from build123d import *

# Parameters (mm, degrees)
PLATE_DEPTH             = 5.08
BOLTHOLES_REACH         = 38.278
SKETCH15_R              = 2.413
UPRIGHT_START           = 67.31
UPRIGHT_DEPTH           = 67.31
UPRIGHT_BOLTHOLES_REACH = 80.133
SKETCH17_R              = 2.54
SKETCH17_R_2            = 2.667
NUT_HOLE_START          = -2.54
NUT_HOLE_DEPTH          = 5.715


with BuildPart() as part:
    # Sketch2 → plate (new body)
    with BuildSketch(Plane(origin=(0, 0, 0), x_dir=(1, 0, 0), z_dir=(0, 1, 0))):
        with BuildLine():
            Line((-15.24, -20.32), (-15.24, -9.8425))
            Line((-15.24, -9.8425), (-3.81, -9.8425))
            Line((-3.81, -9.8425), (-3.81, 9.8425))
            Line((-3.81, 9.8425), (-15.24, 9.8425))
            Line((-15.24, 9.8425), (-15.24, 20.32))
            ThreePointArc((-15.24, 20.32), (25.4, 0), (-15.24, -20.32))
        make_face()
    extrude(amount=PLATE_DEPTH)

    # Sketch15 → boltholes (cut, up to next)
    with BuildSketch(Plane.XZ, mode=Mode.PRIVATE) as boltholes_sk1:
        with Locations(Location((8.89, 13.97, 0), (0, 0, 270))):
            Circle(SKETCH15_R)
    boltholes_tool1 = extrude(boltholes_sk1.sketch, amount=-BOLTHOLES_REACH, mode=Mode.PRIVATE) & part.part
    # Sketch15 → boltholes (cut, up to next)
    with BuildSketch(Plane.XZ, mode=Mode.PRIVATE) as boltholes_sk2:
        with Locations(Location((8.89, -13.97, 0), (0, 0, 270))):
            Circle(SKETCH15_R)
    boltholes_tool2 = extrude(boltholes_sk2.sketch, amount=-BOLTHOLES_REACH, mode=Mode.PRIVATE) & part.part
    add(boltholes_tool1.solids().sort_by_distance((8.89, 0, 13.97))[0], mode=Mode.SUBTRACT)
    add(boltholes_tool2.solids().sort_by_distance((8.89, 0, -13.97))[0], mode=Mode.SUBTRACT)

    # Sketch16 → upright (add)
    with BuildSketch(Plane.XZ.offset(UPRIGHT_START)):
        with BuildLine():
            Line((15.24, 20.32), (15.24, -20.32))
            ThreePointArc((15.24, -20.32), (21.962512448, -12.759625659), (25.200781238, -3.175))
            Line((25.200781238, -3.175), (22.025781238, -3.175))
            Line((22.025781238, -3.175), (22.025781238, 3.175))
            Line((22.025781238, 3.175), (25.200781238, 3.175))
            ThreePointArc((25.200781238, 3.175), (21.962512448, 12.759625659), (15.24, 20.32))
        make_face()
    extrude(amount=-UPRIGHT_DEPTH)

    # Sketch17 → upright_boltholes (cut, up to next)
    with BuildSketch(Plane.ZY.offset(-15.24), mode=Mode.PRIVATE) as upright_boltholes_sk1:
        with Locations((0, -50.8)):
            Circle(SKETCH17_R)
    upright_boltholes_tool1 = extrude(upright_boltholes_sk1.sketch, amount=-UPRIGHT_BOLTHOLES_REACH, mode=Mode.PRIVATE) & part.part
    # Sketch17 → upright_boltholes (cut, up to next)
    with BuildSketch(Plane.ZY.offset(-15.24), mode=Mode.PRIVATE) as upright_boltholes_sk2:
        with Locations((0, -60.96)):
            Circle(SKETCH17_R_2)
    upright_boltholes_tool2 = extrude(upright_boltholes_sk2.sketch, amount=-UPRIGHT_BOLTHOLES_REACH, mode=Mode.PRIVATE) & part.part
    # Sketch17 → upright_boltholes (cut, up to next)
    with BuildSketch(Plane.ZY.offset(-15.24), mode=Mode.PRIVATE) as upright_boltholes_sk3:
        with BuildLine():
            Line((2.54, -12.7), (2.54, -17.78))
            ThreePointArc((2.54, -17.78), (0, -20.32), (-2.54, -17.78))
            Line((-2.54, -17.78), (-2.54, -12.7))
            ThreePointArc((-2.54, -12.7), (0, -10.16), (2.54, -12.7))
        make_face()
    upright_boltholes_tool3 = extrude(upright_boltholes_sk3.sketch, amount=-UPRIGHT_BOLTHOLES_REACH, mode=Mode.PRIVATE) & part.part
    add(upright_boltholes_tool1.solids().sort_by_distance((15.24, -50.8, 0))[0], mode=Mode.SUBTRACT)
    add(upright_boltholes_tool2.solids().sort_by_distance((15.24, -60.96, 0))[0], mode=Mode.SUBTRACT)
    add(upright_boltholes_tool3.solids().sort_by_distance((15.24, -15.24, 0))[0], mode=Mode.SUBTRACT)

    # Sketch18 → nut_hole (cut)
    with BuildSketch(Plane(origin=(22.025781238, 0, 0), x_dir=(0, 0, -1), z_dir=(1, 0, 0)).offset(NUT_HOLE_START)):
        Polygon((0, -66.825878735), (5.08, -63.892939367), (5.08, -58.027060633), (0, -55.094121265), (-5.08, -58.027060633), (-5.08, -63.892939367), align=None)
    extrude(amount=NUT_HOLE_DEPTH, mode=Mode.SUBTRACT)


solid = part.part
Check sheet for the modelled part. Datum: model origin and axes. Units: mm. A direction names the side the tool comes from. Give positions to 0.01 mm unless a question says otherwise; leave off trailing zeros. Write each loop counter-clockwise with the first axis right and the second up, starting at its lowest first coordinate (ties: lowest second). Pieces come first, ordered by that corner, then holes. Notation, with made-up numbers: M 76,17 L 88,17 A13 cw 88,25 Z; hole C -28,3.5 d6. An arc over 180 degrees is marked long. Use one line per item in the form item = value.
(1) Tool access check on faces 4 (the flat face through (-9, 3, -9.842)), 5 (the flat face through (19, -15, 2.54)), 6 (the flat face through (24, 0, 0)). Record the directions out of +Z, -Z, +X, -X, +Y, -Y that give a thin tool (end or side, any length) a straight path to the whole face; none if there is none.
Answer block:
face_4 = -X, +Y, -Y
face_5 = +X, -X
face_6 = +X, -Y
(2) Section check A-A on y = -60.96. Record the boundary of the cut face in (x, z).
Answer block:
outline = M 15.24,-20.32 A25.4 ccw 24.89,-5.08 L 19.49,-5.08 L 19.49,-2.67 L 15.24,-2.67 Z; M 15.24,2.67 L 19.49,2.67 L 19.49,5.08 L 24.89,5.08 A25.4 ccw 15.24,20.32 Z
(3) Depth check by flat-ended pin: P1, Ø9, axis at x = 6, z = 2, coming from the -Y side; P2, Ø4, axis at x = -11, y = 3.5, coming from the -Z side; P3, Ø6, axis at x = 22, y = -62, coming from the +Z side; P4, Ø4.5, axis at x = 8.89, z = 13.97, coming from the +Y side. Enter the tip coordinate at first touch or a pass-through.
Answer block:
P1 = 0
P2 = -23.75
P3 = 16.86
P4 = through
(4) Material ranges on line 1 along Y through (x, z) = (17, 0); line 2 along Z through (x, y) = (8, 3); line 3 along Y through (x, z) = (8.5, -2), recorded low to high.
Answer block:
line_1 = -67.31 to -63.63, -58.29 to -53.34, -48.26 to -20.32, -10.16 to 5.08
line_2 = -24.11 to -16.21, -11.73 to 11.73, 16.21 to 24.11
line_3 = 0 to 5.08
(5) Section check D-D on y = -50.8. Record the boundary of the cut face in (x, z) (3 decimals), plus the area to 3 significant figures.
Answer block:
outline = M 15.24,-20.32 A25.4 ccw 25.201,-3.175 L 22.026,-3.175 L 22.026,-2.54 L 15.24,-2.54 Z; M 15.24,2.54 L 22.026,2.54 L 22.026,3.175 L 25.201,3.175 A25.4 ccw 15.24,20.32 Z
area = 233 mm2
(6) Section check B-B on z = -13.97. Record the boundary of the cut face in (x, y).
Answer block:
outline = M -15.24,0 L 6.48,0 L 6.48,5.08 L -15.24,5.08 Z; M 11.3,0 L 15.24,0 L 15.24,-67.31 L 21.21,-67.31 L 21.21,5.08 L 11.3,5.08 Z
(7) Draft check along Y on faces 1 (the flat face through (0, 0, 0)), 2 (the flat face through (22.026, -29, 0)), 3 (the flat face through (21.668, -65.054, -3.069)). Enter one of: pulls with the +Y half, pulls with the -Y half, needs draft (parallel to the pull), parting line crosses it, or undercut.
Answer block:
face_1 = pulls with the -Y half
face_2 = needs draft
face_3 = undercut
(8) Section check C-C on x = 10.5. Record the boundary of the cut face in (y, z).
Answer block:
outline = M 0,-23.13 L 5.08,-23.13 L 5.08,-15.77 L 0,-15.77 Z; M 0,-12.17 L 5.08,-12.17 L 5.08,12.17 L 0,12.17 Z; M 0,15.77 L 5.08,15.77 L 5.08,23.13 L 0,23.13 Z
